Can you work these out from the model? Positions are in its coordinate system, mm. A direction names the side the tool comes from. Coordinates: 2 decimals unless noted, no trailing zeros. Order: outer loops, then holes, each group sorted by start corner. A loop starts at its lowest first (then second) coordinate and runs counter-clockwise, first axis right, second up. Notation, with made-up numbers: (75.25, 76.5) -> (111.25, 76.5) arc R22 cw to (111.25, 112.5) -> close; hole circle Ø2 at (34, 21). An arc over 180 degrees is marked (long way). Use a Markdown table: item, result. Add a question column.
1. For faces 1 (the flat face through (67.5, 38, 2)), 2 (the cylindrical face through (-33, 16.07, 2.54)), 3 (the flat face through (-76, -15, 2)), 4 (the flat face through (-76, 15, 2)), which set-ups out of +Z, -Z, +X, -X, +Y, -Y let a thin tool reach every point of the face, with its end or its side?
2. Suppose I cut it at B-B, the plane z = 1.6. State how many separate pieces and enclosed holes the cut face has, then the cut area to 3 significant figures.
3. Suppose I cut it at A-A, the plane x = -25. List the corners of the cut face in (y, z) for me, then the cut area to 3 significant figures.
4. We'd pull the mould along Y, two halves only. Please class faces 5 (the flat face through (-53.5, 33, 2)), 6 (the flat face through (37, 1, 5)), 7 (the flat face through (76, 15, 2)): pulls with the +Y half, pulls with the -Y half, needs draft (parallel to the pull), parting line crosses it, or undercut.
5. For pin 1 Ø8 at (x, y) = (-42.31, -7.3) entering from +Z; pin 2 Ø3 at (x, y) = (-40, 60.5) entering from -Z; pin 3 Ø2.5 at (y, z) = (-41, 3) entering from +X, each with a flat end and sliding along its axis, tell me the tip position at first contact or that it passes through.
6. If I drill on line 1 along X through (y, z) = (60.5, 3.2); line 2 along X through (y, z) = (-40, 3.55), over which ranges is the centre line in solid material (lowest first)? Write a range as from..to.
```python
from build123d import *

# Parameters (mm, degrees)
F1_DEPTH       = 5
F2_D           = 2.5
F2_CSINK_D     = 4
F2_CSINK_ANGLE = 90
F3_R           = 5
F4_R           = 5
F6_D           = 6
F6_DEPTH       = 12
F6_CSINK_D     = 10
F6_CSINK_ANGLE = 90
F6_TIP         = 1.8025818571


with BuildPart() as f1:
    # F0 (on Top) → F1 (new body)
    with BuildSketch(Plane.XY):
        Polygon((-67.5, -67.5), (67.5, -67.5), (67.5, -15), (67.5, 0), (67.5, 15), (67.5, 67.5), (-67.5, 67.5), (-67.5, 15), (-67.5, 0), (-67.5, -15), align=None)
        Polygon((-53.5, 17.5), (-53.5, 53.5), (53.5, 53.5), (53.5, 17.5), (53.5, 0), (53.5, -17.5), (53.5, -53.5), (-53.5, -53.5), (-53.5, -17.5), align=None, mode=Mode.SUBTRACT)
        Polygon((-31.5, 17.5), (-53.5, 17.5), (-53.5, -17.5), (-31.5, -17.5), (-31.5, 0), align=None)
        Polygon((53.5, 0), (53.5, 17.5), (33.5, 17.5), (33.5, 0), (33.5, -17.5), (53.5, -17.5), align=None)
        Polygon((-85, -15), (-67.5, -15), (-67.5, 0), (-67.5, 15), (-85, 15), (-85, 0), align=None)
        Polygon((67.5, 0), (67.5, -15), (85, -15), (85, 0), (85, 15), (67.5, 15), align=None)
    extrude(amount=F1_DEPTH)

    # F2 (through all)
    with Locations(Plane(origin=(0, 0, 0), x_dir=(1, 0, 0), z_dir=(0, 0, -1))):
        with Locations((-60.5, 0), (-60.5, 40), (-60.5, -40), (-40, -60.5), (0, -60.5), (40, -60.5), (60.5, -40), (60.5, 0), (60.5, 40), (40, 60.5), (0, 60.5), (-40, 60.5), (-80, 10), (-80, -10), (80, 10), (80, -10)):
            CounterSinkHole(F2_D / 2, F2_CSINK_D / 2, counter_sink_angle=F2_CSINK_ANGLE)

    # F3
    f3_edges = [f1.edges().sort_by_distance(p)[0] for p in [
        (-31.5, 17.5, 2.5),
        (33.5, -17.5, 2.5),
        (33.5, 17.5, 2.5),
        (-67.5, 67.5, 2.5),
        (67.5, 67.5, 2.5),
        (67.5, -67.5, 2.5),
        (-31.5, -17.5, 2.5),
        (-67.5, -67.5, 2.5),
    ]]
    fillet(f3_edges, radius=F3_R)

    # F4
    f4_edges = [f1.edges().sort_by_distance(p)[0] for p in [
        (-53.5, -53.5, 2.5),
        (-53.5, 53.5, 2.5),
        (53.5, -53.5, 2.5),
        (53.5, 53.5, 2.5),
    ]]
    fillet(f4_edges, radius=F4_R)

    # F6
    with Locations(Plane.XY.offset(5)):
        with Locations((-42.3126109545, 7.2952777508), (-42.3126109545, -7.2952777508), (42.3126109545, 7.2952777508), (42.3126109545, -7.2952777508)):
            CounterSinkHole(F6_D / 2, F6_CSINK_D / 2, depth=F6_DEPTH, counter_sink_angle=F6_CSINK_ANGLE)
            with Locations((0, 0, -(F6_DEPTH + F6_TIP / 2))):  # 118° drill point
                Cone(0, F6_D / 2, F6_TIP, mode=Mode.SUBTRACT)


solid = f1.part
```
Worked out:
| question | item | result |
|---|---|---|
| 1 | face 1 | +Z, -Z, +X, +Y |
| 1 | face 2 | +Z, -Z |
| 1 | face 3 | +Z, -Z, -X, -Y |
| 1 | face 4 | +Z, -Z, -X, +Y |
| 2 | separate pieces | 1 |
| 2 | enclosed holes | 21 |
| 2 | area | 9,080 mm² |
| 3 | outline | (-67.5, 0) -> (-53.5, 0) -> (-53.5, 5) -> (-67.5, 5) -> close; (53.5, 0) -> (67.5, 0) -> (67.5, 5) -> (53.5, 5) -> close |
| 3 | area | 140 mm² |
| 4 | face 5 | undercut |
| 4 | face 6 | needs draft |
| 4 | face 7 | pulls with the +Y half |
| 5 | pin 1 | stops at z = 4.01 |
| 5 | pin 2 | stops at z = 0.5 |
| 5 | pin 3 | stops at x = 67.5 |
| 6 | line 1 | x = -67.5..-41.25, -38.75..-1.25, 1.25..38.75, 41.25..67.5 |
| 6 | line 2 | x = -67.5..-61.75, -59.25..-53.5, 53.5..59.25, 61.75..67.5 |
